```python
from build123d import *

# Parameters (mm, degrees)
SKETCH1_W               = 80
SKETCH1_H               = 70
BOSS_EXTRUDE1_DEPTH     = 15
BOSS_EXTRUDE2_DEPTH     = 70
SKETCH3_W               = 20
SKETCH3_H               = 70
BOSS_EXTRUDE3_DEPTH     = 15
SKETCH4_W               = 10
SKETCH4_H               = 15
BOSS_EXTRUDE4_DEPTH     = 30
BOSS_EXTRUDE5_DEPTH     = 30
CUT_EXTRUDE1_DEPTH      = 15
CUT_EXTRUDE2_START      = 15
CUT_EXTRUDE2_DEPTH      = 60
CUT_EXTRUDE3_DEPTH      = 116.758369028
CUT_EXTRUDE3_DEPTH_BACK = 116.758369028
CUT_EXTRUDE4_DEPTH      = 116.758369028
CUT_EXTRUDE4_DEPTH_BACK = 116.758369028
SKETCH9_W               = 40
SKETCH9_H               = 40


with BuildPart() as part:
    # Sketch1 → Boss-Extrude1 (new body)
    with BuildSketch(Plane(origin=(0, 0, 0), x_dir=(1, 0, 0), z_dir=(0, 1, 0))):
        with Locations((0, -35)):
            Rectangle(SKETCH1_W, SKETCH1_H)
    extrude(amount=BOSS_EXTRUDE1_DEPTH)

    # Sketch2 → Boss-Extrude2 (add)
    with BuildSketch(Plane.XY):
        with BuildLine():
            Line((-30, 15), (30, 15))
            Line((30, 15), (30, 28.542486889))
            ThreePointArc((30, 28.542486889), (37.416573868, 40.857864376), (40, 55))
            Line((40, 55), (-40, 55))
            ThreePointArc((-40, 55), (-37.416573868, 40.857864376), (-30, 28.542486889))
            Line((-30, 28.542486889), (-30, 15))
        make_face()
    extrude(amount=BOSS_EXTRUDE2_DEPTH)

    # Sketch3 → Boss-Extrude3 (add)
    with BuildSketch(Plane(origin=(0, 0, 0), x_dir=(1, 0, 0), z_dir=(0, 1, 0))):
        with Locations((-50, -35)):
            Rectangle(SKETCH3_W, SKETCH3_H)
    boss_extrude3 = extrude(amount=BOSS_EXTRUDE3_DEPTH)

    # Sketch4 → Boss-Extrude4 (add)
    with BuildSketch(Plane.XY):
        with Locations((-35, 62.5)):
            Rectangle(SKETCH4_W, SKETCH4_H)
    boss_extrude4 = extrude(amount=BOSS_EXTRUDE4_DEPTH)

    # Sketch5 → Boss-Extrude5 (add)
    with BuildSketch(Plane.XY):
        Polygon((-60, 15), (-40, 70), (-40, 55), (-30, 55), (-30, 15), align=None)
    boss_extrude5 = extrude(amount=BOSS_EXTRUDE5_DEPTH)

    # Sketch6 → Cut-Extrude1 (cut)
    with BuildSketch(Plane(origin=(0, 0, 0), x_dir=(1, 0, 0), z_dir=(0, 1, 0))):
        Polygon((-60, -20), (-40, -70), (-60, -70), align=None)
    cut_extrude1 = extrude(amount=CUT_EXTRUDE1_DEPTH, mode=Mode.SUBTRACT)

    # Sketch7 → Cut-Extrude2 (cut)
    with BuildSketch(Plane(origin=(0, 0, 0), x_dir=(1, 0, 0), z_dir=(0, 1, 0)).offset(CUT_EXTRUDE2_START)):
        Polygon((-60, -20), (-40, -30), (-60, -30), align=None)
    cut_extrude2 = extrude(amount=CUT_EXTRUDE2_DEPTH, mode=Mode.SUBTRACT)

    # Mirror1: Boss-Extrude3, Boss-Extrude4, Boss-Extrude5, Cut-Extrude1, Cut-Extrude2 across plane
    add(boss_extrude3.mirror(Plane(origin=(0, 0, 0), x_dir=(0, 0, 1), z_dir=(1, 0, 0))))
    add(boss_extrude4.mirror(Plane(origin=(0, 0, 0), x_dir=(0, 0, 1), z_dir=(1, 0, 0))))
    add(boss_extrude5.mirror(Plane(origin=(0, 0, 0), x_dir=(0, 0, 1), z_dir=(1, 0, 0))))
    add(cut_extrude1.mirror(Plane(origin=(0, 0, 0), x_dir=(0, 0, 1), z_dir=(1, 0, 0))), mode=Mode.SUBTRACT)
    add(cut_extrude2.mirror(Plane(origin=(0, 0, 0), x_dir=(0, 0, 1), z_dir=(1, 0, 0))), mode=Mode.SUBTRACT)

    # Sketch8 → Cut-Extrude3 (cut, two sides: drawn at the far end of the back side and taken through both)
    with BuildSketch(Plane.XY.offset(-CUT_EXTRUDE3_DEPTH_BACK)):
        with BuildLine():
            Line((-30, 72), (-30, 55))
            ThreePointArc((-30, 55), (0, 25), (30, 55))
            Line((30, 55), (30, 72))
            Line((30, 72), (-30, 72))
        make_face()
    extrude(amount=CUT_EXTRUDE3_DEPTH + CUT_EXTRUDE3_DEPTH_BACK, mode=Mode.SUBTRACT)

    # Sketch9 → Cut-Extrude4 (cut, two sides: drawn at the far end of the back side and taken through both)
    with BuildSketch(Plane(origin=(0, 0, 0), x_dir=(1, 0, 0), z_dir=(0, 1, 0)).offset(-CUT_EXTRUDE4_DEPTH_BACK)):
        with Locations((0, -30)):
            Rectangle(SKETCH9_W, SKETCH9_H)
    extrude(amount=CUT_EXTRUDE4_DEPTH + CUT_EXTRUDE4_DEPTH_BACK, mode=Mode.SUBTRACT)


solid = part.part
```
Input: part model. Units: mm. Frame: model coordinates. A direction names the side the tool comes from. Coordinates: 2 decimals unless noted, no trailing zeros. Order: outer loops, then holes, each group sorted by start corner. A loop starts at its lowest first (then second) coordinate and runs counter-clockwise, first axis right, second up. Notation, with made-up numbers: (86.5, 54) - (144.5, 54) arc R27 ccw to (144.5, 89) - close; hole circle Ø5 at (64, 87.5). An arc over 180 degrees is marked (long way). Put each result on its own line as item: value.
1. Cut plane D-D on y = 10. Return the cut outline in (x, z), then the cut area to 3 significant figures.
Report:
outline: (-60, 0) - (60, 0) - (60, 20) - (40, 70) - (-40, 70) - (-60, 20) - close; hole (-20, 10) - (20, 10) - (20, 50) - (-20, 50) - close
area: 5,800 mm2
2. Reachability of faces 1 (the face through (-41, 15, 45)), 2 (the face through (-20, 16, 30)), 3 (the face through (35, 63, 30)), 4 (the face through (37.345, 40.669, 49.72)), 5 (the face through (-30, 62, 15)) from +Z, -Z, +X, -X, +Y, -Y: full face, straight path, thin tool, end or side. Return the list, or none.
Report:
face 1: +Z, -X
face 2: +Y, -Y
face 3: +Z, +X, -X, +Y
face 4: +Z, +X
face 5: +Z, -Z, +Y
3. Cut plane B-B on x = 0. Return the cut outline in (y, z), then the cut area to 3 significant figures.
Report:
outline: (0, 0) - (25, 0) - (25, 10) - (0, 10) - close; (0, 50) - (25, 50) - (25, 70) - (0, 70) - close
area: 750 mm2
4. Line query: line 1 along Z through (x, y) = (3, 7); line 2 along X through (y, z) = (15, 11); line 3 along X through (y, z) = (38, 45). Output: solid intervals per line, ascending.
Report:
line 1: z = 0 to 10, 50 to 70
line 2: x = -60 to -20, 20 to 60
line 3: x = -36.21 to -24.72, 24.72 to 36.21
5. Cut plane C-C on y = 42. Return the cut outline in (x, z).
Report:
outline: (-50.18, 0) - (-27.04, 0) - (-27.04, 70) - (-37.83, 70) - (-37.83, 30) - (-40, 30) - (-50.18, 24.91) - close; (27.04, 0) - (50.18, 0) - (50.18, 24.91) - (40, 30) - (37.83, 30) - (37.83, 70) - (27.04, 70) - close
6. Draft query along X for faces 6 (the face through (30, 62, 15)), 7 (the face through (-50.14, 42.12, 11.46)), 8 (the face through (-36, 26, 30)). Return one class per face: pulls with the +X half, pulls with the -X half, needs draft (parallel to the pull), parting line crosses it, or undercut.
Report:
face 6: undercut
face 7: pulls with the -X half
face 8: needs draft
7. Contact query for flat-ended pins moving along their axis: pin 1 Ø10 at (x, z) = (-40.5, 51) entering from +Y; pin 2 Ø3 at (y, z) = (28, 16.5) entering from +X; pin 3 Ø15 at (x, z) = (50.5, 43.5) entering from +Y. Output: stop coordinate, or through.
Report:
pin 1: stops at y = 55
pin 2: stops at x = 55.82
pin 3: stops at y = 15
8. Cut plane A-A on z = 48.5. Return the cut outline in (x, y), then the cut area to 3 significant figures.
Report:
outline: (-48.6, 0) - (-20, 0) - (-20, 32.64) arc R30 cw to (-30, 55) - (-40, 55) arc R40 ccw to (-30, 28.54) - (-30, 15) - (-48.6, 15) - close; (20, 0) - (48.6, 0) - (48.6, 15) - (30, 15) - (30, 28.54) arc R40 ccw to (40, 55) - (30, 55) arc R30 cw to (20, 32.64) - close
area: 1,710 mm2
